Build history of the part. All positions in model axes, mm. Give positions to 0.01 mm unless a question says otherwise; leave off trailing zeros. Loops run counter-clockwise (first coordinate to the right, second up) from the corner with the lowest first, then second, coordinate; pieces in that order, holes last. Notation, with made-up numbers: (87, 56.25) -> (107, 56.25) arc R23 cw to (107, 88.25) -> close; hole circle Ø7 at (-39, 5). An arc over 180 degrees is marked (long way). Answer as a JSON object with one key per item and string values. Group by question number.
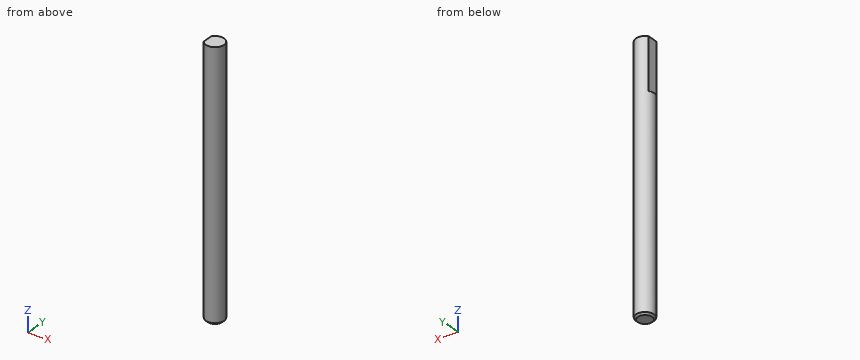
from build123d import *

# Parameters (mm, degrees)
CROQUIS1_R              = 2.5
SALIENTE_EXTRUIR1_DEPTH = 71
CUT_EXTRUDE1_DEPTH      = 14
CHAMFER1_SIZE           = 0.5


with BuildPart() as part:
    # Croquis1 → Saliente-Extruir1 (new body)
    with BuildSketch(Plane.XY):
        Circle(CROQUIS1_R)
    extrude(amount=SALIENTE_EXTRUIR1_DEPTH)

    # Sketch1 → Cut-Extrude1 (cut)
    with BuildSketch(Plane.XY.offset(71)):
        with BuildLine():
            Line((-2.05, 1.430908802), (-2.05, -1.430908802))
            ThreePointArc((-2.05, -1.430908802), (-2.5, 0), (-2.05, 1.430908802))
        make_face()
    extrude(amount=-CUT_EXTRUDE1_DEPTH, mode=Mode.SUBTRACT)

    # Chamfer1
    chamfer1_edges = [part.edges().sort_by_distance(p)[0] for p in [
        (-2.5, 0, 0),
    ]]
    chamfer(chamfer1_edges, length=CHAMFER1_SIZE)


solid = part.part
(1) Pin check, flat tips, straight feed: pin 1 (3 mm diameter, centred on x = 0.5, y = -1.5, fed in from -Z); pin 2 (1 mm diameter, centred on y = -2, z = 33.5, fed in from -X); pin 3 (2.5 mm diameter, centred on y = -0.5, z = 61, fed in from -X); pin 4 (1 mm diameter, centred on y = -2, z = 30.5, fed in from +X). Stop position of each tip, or through.
(2) Probe line 1 along X through (y, z) = (-1.5, 39.5); line 2 along Y through (x, z) = (0.1, 7); line 3 along X through (y, z) = (0.2, 65). List the from-to ranges inside material, lowest first. Write a range as [from, to].
(3) Saw through at B-B on z = 61.5. List the corners of the cut face in (x, y), plus the area to 3 significant figures.
(4) Saw through at C-C on z = 16.5. List the corners of the cut face in (x, y), plus the area to 3 significant figures.
(5) Saw through at A-A on y = 0. List the corners of the cut face in (x, z), plus the area to 3 significant figures.
Calculated:
{
 "1": {"pin 1": "stops at z = 0", "pin 2": "stops at x = -2", "pin 3": "stops at x = -2.05", "pin 4": "stops at x = 2"},
 "2": {"line 1": "x = [-2, 2]", "line 2": "y = [-2.5, 2.5]", "line 3": "x = [-2.05, 2.49]"},
 "3": {"outline": "(-2.05, -1.43) arc R2.5 ccw (long way) to (-2.05, 1.43) -> close", "area": "18.8 mm^2"},
 "4": {"outline": "circle Ø5 at (0, 0)", "area": "19.6 mm^2"},
 "5": {"outline": "(-2.5, 0.5) -> (-2, 0) -> (2, 0) -> (2.5, 0.5) -> (2.5, 71) -> (-2.05, 71) -> (-2.05, 57) -> (-2.5, 57) -> close", "area": "348 mm^2"}
}
